Part model, mm, in its own coordinate system. A direction names the side the tool comes from. Coordinates: 2 decimals unless noted, no trailing zeros. Write each loop counter-clockwise with the first axis right and the second up, starting at its lowest first coordinate (ties: lowest second). Pieces come first, ordered by that corner, then holes. Notation, with made-up numbers: (-40, 80) - (-29, 80) arc R24 cw to (-29, 104) - close; hole circle Ø11 at (85, 81.5). An arc over 180 degrees is marked (long way). Write each question's results on one line, items separated by ' | '.
from build123d import *

# Parameters (mm, degrees)
SKETCH1_R          = 44.49044586
EXTRUDE1_DEPTH     = 280
FILLET1_R          = 25.4
SKETCH3_W          = 20
SKETCH3_H          = 10
CUT_EXTRUDE1_DEPTH = 7.62
SKETCH4_R          = 19.05
CUT_EXTRUDE2_DEPTH = 7.62


with BuildPart() as part:
    # Sketch1 → Extrude1 (new body)
    with BuildSketch(Plane.XY):
        Circle(SKETCH1_R)
    extrude(amount=EXTRUDE1_DEPTH)

    # Fillet1
    fillet1_edges = [part.edges().sort_by_distance(p)[0] for p in [
        (-44.49044586, 0, 0),
        (-44.49044586, 0, 280),
    ]]
    fillet(fillet1_edges, radius=FILLET1_R)

    # Sketch3 → Cut-Extrude1 (cut)
    with BuildSketch(Plane(origin=(0, 0, 0), x_dir=(-1, 0, 0), z_dir=(0, 0, -1))):
        Rectangle(SKETCH3_W, SKETCH3_H)
    extrude(amount=-CUT_EXTRUDE1_DEPTH, mode=Mode.SUBTRACT)

    # Sketch4 → Cut-Extrude2 (cut)
    with BuildSketch(Plane.XY.offset(280)):
        Circle(SKETCH4_R)
    extrude(amount=-CUT_EXTRUDE2_DEPTH, mode=Mode.SUBTRACT)


solid = part.part
(1) 3-axis set-ups, long thin cutter, end or side, ignore diameter. For faces 1 (the flat face through (0, -5, 4)), 2 (the flat face through (0, 0, 272.38)): which of +Z, -Z, +X, -X, +Y, -Y reach the whole face in a straight line?
Return value:
face 1: -Z | face 2: +Z
(2) Flat gauge pins, fed straight in: P1, Ø4, axis at x = -30.5, z = 34.5, coming from the -Y side; P2, Ø8.5, axis at y = 0, z = 4.5, coming from the -X side; P3, Ø1, axis at x = -3, z = 76.5, coming from the -Y side. Where does each tip first touch, or does it go through?
Return value:
P1: stops at y = -34.16 | P2: stops at x = -38.27 | P3: stops at y = -44.42
(3) Two-plate mould, pull along Y, no slides. Class faces 3 (the flat face through (0, -8, 0)), 4 (the cylindrical face through (-35.306, -27.072, 138.396)), 5 (the cylindrical face through (-15.12, -11.59, 276.24)): released by +Y, released by -Y, zero draft, split by the parting line, or undercut.
Return value:
face 3: zero draft | face 4: split by the parting line | face 5: undercut
(4) Saw through at A-A on z = 150. Write the cut outline in (x, y).
Return value:
outline: circle Ø88.98 at (0, 0)
(5) Wall check: line 1 (Z direction, x = -13.5, y = -11.5); line 2 (Y direction, x = 0, z = 199); line 3 (Y direction, x = 0, z = 277). Give the ranges that are in metal, low to high. Write a range as from..to.
Return value:
line 1: z = 0..272.38 | line 2: y = -44.49..44.49 | line 3: y = -31.07..-19.05, 19.05..31.07
